```python
from build123d import *

# Parameters (mm, degrees)
SKETCH1_R           = 1.5
BOSS_EXTRUDE1_DEPTH = 10
SKETCH3_R           = 4
CUT_EXTRUDE2_DEPTH  = 6
SHELL11_T           = -0.5


# Read off the part's stored shape, not the designer's step: Dome1
with BuildPart() as part:
    # Sketch1 → Boss-Extrude1 (new body)
    with BuildSketch(Plane.XY):
        Circle(SKETCH1_R)
    extrude(amount=BOSS_EXTRUDE1_DEPTH)

    # Dome1 outline → Dome1 (revolve)
    with BuildSketch(Plane.XZ):
        with BuildLine():
            Line((0, 2e-09), (0, -6))
            ThreePointArc((0, -6), (3.09232922, -3.585582304), (1.499999999, 1e-09))
            Line((1.499999999, 1e-09), (0, 2e-09))
        make_face()
    revolve(axis=Axis((0, 0, 0), (0, 0, 1)))

    # Sketch3 → Cut-Extrude2 (cut)
    with BuildSketch(Plane.XY.offset(-10)):
        Circle(SKETCH3_R)
    extrude(amount=CUT_EXTRUDE2_DEPTH, mode=Mode.SUBTRACT)

    # Shell11
    shell11_openings = [part.faces().sort_by_distance(p)[0] for p in [
        (1e-09, 0, -4),
    ]]
    offset(amount=SHELL11_T, openings=shell11_openings, kind=Kind.INTERSECTION)


solid = part.part
```
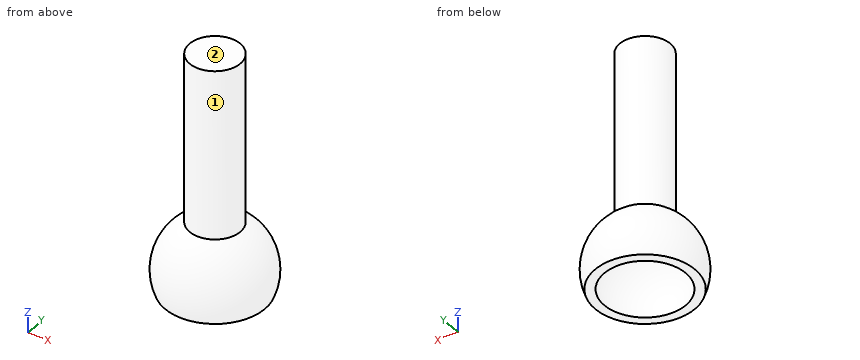
Check sheet for the modelled part. Datum: model origin and axes. Units: mm. Face numbers are marked on the shaded views. Round coordinates to 2 decimals unless told otherwise and drop trailing zeros. Loops run counter-clockwise (first coordinate to the right, second up) from the corner with the lowest first, then second, coordinate; pieces in that order, holes last. Notation, with made-up numbers: (61.25, 25.25) - (95.25, 25.25) arc R25 cw to (95.25, 42.25) - close; hole circle Ø1 at (-32.75, 54.25). An arc over 180 degrees is marked (long way). Write item = value, one per line. Start each with the question number.
Q1. Thickness scan on L1, parallel to Y at x = 0, z = 4.75; L2, parallel to X at y = 1.5, z = -1.5; L3, parallel to X at y = -0.75, z = 0.5. Record the ranges inside material, lowest first.
Q2. Release check for a two-part mould opening along X. For the marked faces 1 and 2 record: pulls with the +X half, pulls with the -X half, needs draft (parallel to the pull), parting line crosses it, or undercut.
Q3. Section check D-D (z = -1). Record the boundary of the cut face in (x, y).
Q4. Section check C-C (x = 0). Record the boundary of the cut face in (y, z) (1 decimal).
Q5. Depth check by flat-ended pin: P1, Ø1.5, axis at x = -0.5, z = 1.5, coming from the +Y side; P2, Ø3, axis at x = 0, y = 0, coming from the -Z side; P3, Ø2, axis at x = 1.5, z = 8, coming from the +Y side. Enter the tip coordinate at first touch or a pass-through.
Q6. Section check B-B (z = 0.5). Record the boundary of the cut face in (x, y), plus the area to 3 significant figures.
Q7. Section check A-A (y = 0.5). Record the boundary of the cut face in (x, z), plus the area to 3 significant figures.
Derived:
q1.L1 = -1.5 to -1, 1 to 1.5
q1.L2 = -2.49 to -1.8, 1.8 to 2.49
q1.L3 = -1.3 to -0.66, 0.66 to 1.3
q2.face_1 = parting line crosses it
q2.face_2 = needs draft
q3.outline = circle Ø5.24 at (0, 0); hole circle Ø3.97 at (0, 0)
q4.outline = (-3, -4) - (-2.4, -4) arc R2.7 cw to (-1, -0.3) - (-1, 9.5) - (1, 9.5) - (1, -0.3) arc R2.7 cw to (2.4, -4) - (3, -4) arc R3.2 ccw to (1.5, 0) - (1.5, 10) - (-1.5, 10) - (-1.5, 0) arc R3.2 ccw to start
q5.P1 = 1.5
q5.P2 = -0.58
q5.P3 = 1.41
q6.outline = circle Ø3 at (0, 0); hole circle Ø2 at (0, 0)
q6.area = 3.93 mm^2
q7.outline = (-2.92, -4) - (-2.36, -4) arc R2.64 cw to (-0.87, -0.32) - (-0.87, 9.5) - (0.87, 9.5) - (0.87, -0.32) arc R2.64 cw to (2.36, -4) - (2.92, -4) arc R3.15 ccw to (1.41, 0) - (1.41, 10) - (-1.41, 10) - (-1.41, 0) arc R3.15 ccw to start
q7.area = 16.7 mm^2
